Geometry check sheet. Reference: drawing and pictorial views, mm from the part's lowest x, y, z. A direction names the side the tool comes from. Round coordinates to 2 decimals unless told otherwise and drop trailing zeros. Order: outer loops, then holes, each group sorted by start corner. A loop starts at its lowest first (then second) coordinate and runs counter-clockwise, first axis right, second up.
(1) Thickness scan on probe 1 along Y at (x, z) = (29, 44.5); probe 2 along X at (y, z) = (26, 34.5) (1 decimal); probe 3 along Y at (x, z) = (4, 24) (1 decimal). Record the ranges inside material, lowest first.
(2) Sectioned sample at B-B, the plane z = 34. Enter the section's corners in (x, y) (1 decimal), and give its area (3 significant figures).
(3) Tool access check on the marked faces 4 and 5. Record the directions out of +Z, -Z, +X, -X, +Y, -Y that give a thin tool (end or side, any length) a straight path to the whole face; none if there is none.
(4) Sectioned sample at A-A, the plane z = 12. Enter the section's corners in (x, y) (1 decimal).
(5) Depth check by flat-ended pin: pin 1 (10 mm diameter, centred on y = 14.5, z = 15, fed in from -X); pin 2 (5.5 mm diameter, centred on x = 29.09, y = 29.09, fed in from +Z); pin 3 (10 mm diameter, centred on x = 20.5, y = 13, fed in from +Z); pin 4 (2.5 mm diameter, centred on x = 29.09, y = 29.09, fed in from -Z). Enter the tip coordinate at first touch or a pass-through.
(6) Mould release check, pull along X, two halves, no side actions. Record for the marked faces 1, 2 and 3: released by +X, released by -X, zero draft, split by the parting line, or undercut.
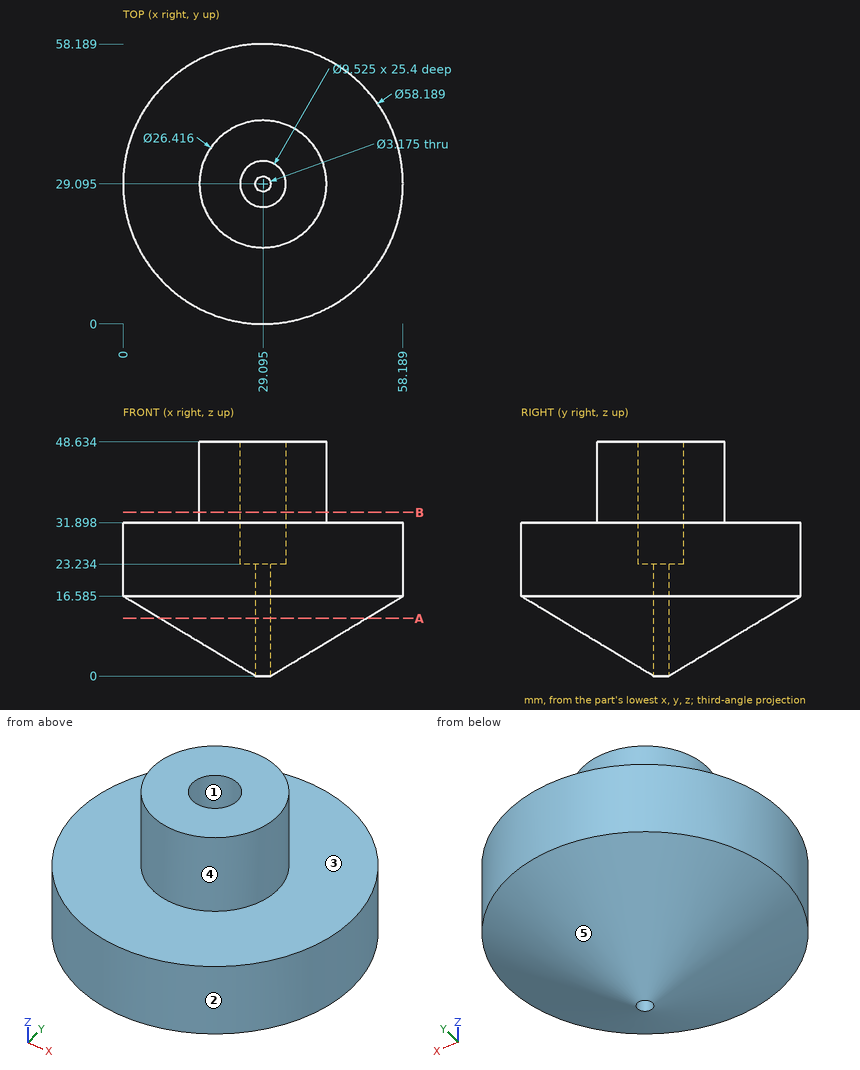
Derived:
1. probe 1: y = 15.89 to 24.33, 33.86 to 42.3
1. probe 2: x = 16.3 to 25.5, 32.7 to 41.9
1. probe 3: y = 14.4 to 43.8
2. outline: circle Ø26.4 at (29.1, 29.1); hole circle Ø9.5 at (29.1, 29.1)
2. area: 477 mm2
3. face 4: +Z
3. face 5: -Z
4. outline: circle Ø43 at (29.1, 29.1); hole circle Ø3.2 at (29.1, 29.1)
5. pin 1: stops at x = 1.72
5. pin 2: stops at z = 23.23
5. pin 3: stops at z = 31.9
5. pin 4: passes through
6. face 1: undercut
6. face 2: split by the parting line
6. face 3: zero draft
